Check sheet for the drawn part. Datum: minimum x, y, z corner. Units: mm. A direction names the side the tool comes from. Round coordinates to 2 decimals unless told otherwise and drop trailing zeros. Order: outer loops, then holes, each group sorted by start corner. A loop starts at its lowest first (then second) coordinate and runs counter-clockwise, first axis right, second up. Notation, with made-up numbers: (61.5, 15.5) -> (95.5, 15.5) arc R20 cw to (95.5, 36.5) -> close; hole circle Ø7 at (11.25, -2). An arc over 180 degrees is marked (long way). Answer as a JSON object with one key per item and string values. Group by question number.
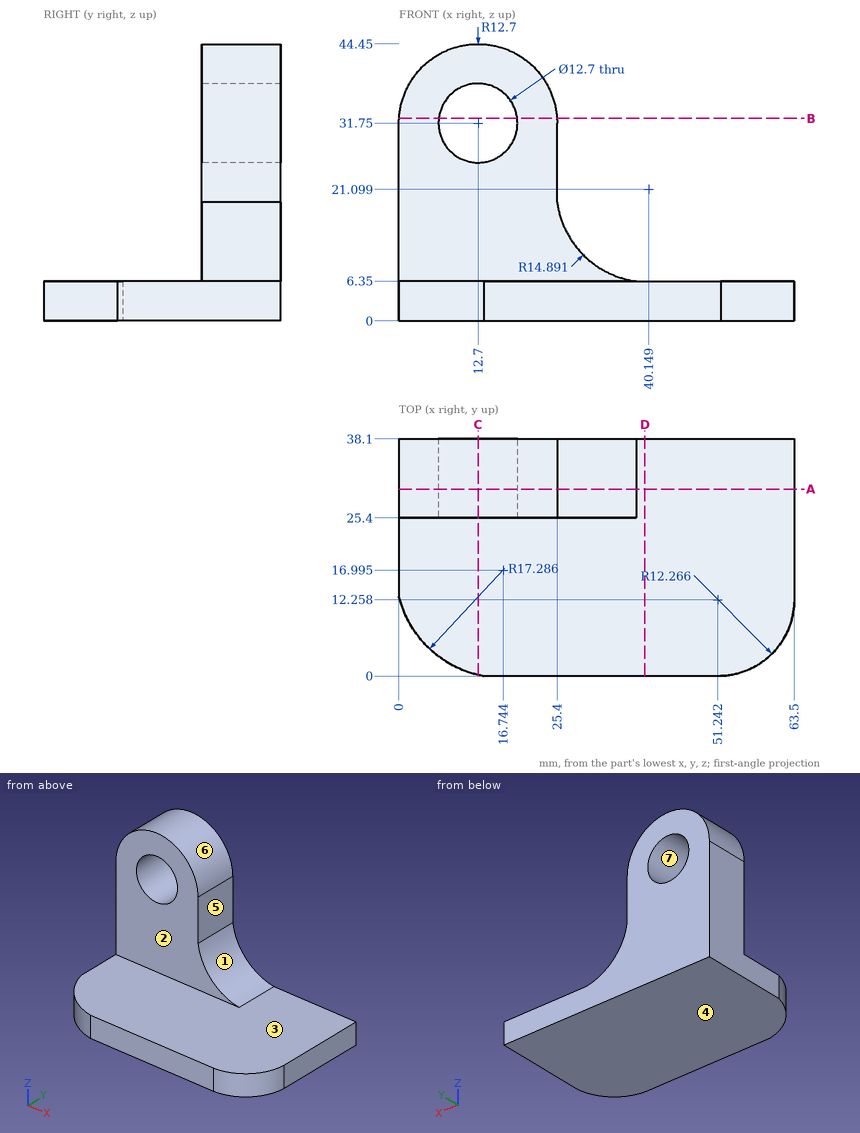
Item 1: Depth check by flat-ended pin: pin 1 Ø20.5 at (x, z) = (12.7, 31.75) entering from +Y; pin 2 Ø3 at (x, z) = (7.5, 31.5) entering from -Y; pin 3 Ø11.5 at (x, y) = (34, 18) entering from +Z; pin 4 Ø14 at (y, z) = (34, 26.5) entering from +X. Enter the tip coordinate at first touch or a pass-through.
Item 2: Mould release check, pull along Z, two halves, no side actions. Record for the marked faces 4, 5, 6 and 7: pulls with the +Z half, pulls with the -Z half, needs draft (parallel to the pull), parting line crosses it, or undercut.
Item 3: Thickness scan on L1, parallel to Z at x = 12.7, y = 29.5; L2, parallel to Z at x = 57, y = 30; L3, parallel to X at y = 30, z = 31 (1 decimal). Record the ranges inside material, lowest first.
Item 4: Sectioned sample at D-D, the plane x = 39.5. Enter the section's corners in (y, z), then the cut area to 3 significant figures.
Item 5: Sectioned sample at A-A, the plane y = 30. Enter the section's corners in (x, z), then the cut area to 3 significant figures.
Item 6: Set-up check for the marked faces 1, 2 and 3: record each of +Z, -Z, +X, -X, +Y, -Y from which the full face is reachable in a straight line by a thin tool's end or side.
Item 7: Sectioned sample at C-C, the plane x = 12.7. Enter the section's corners in (y, z), then the cut area to 3 significant figures.
Item 8: Sectioned sample at B-B, the plane z = 32.5. Enter the section's corners in (x, y) (1 decimal), then the cut area to 3 significant figures.
Result:
{
 "1": {"pin 1": "stops at y = 38.1", "pin 2": "stops at y = 25.4", "pin 3": "stops at z = 6.35", "pin 4": "stops at x = 25.4"},
 "2": {"face 4": "pulls with the -Z half", "face 5": "needs draft", "face 6": "pulls with the +Z half", "face 7": "undercut"},
 "3": {"L1": "z = 0 to 25.4, 38.1 to 44.45", "L2": "z = 0 to 6.35", "L3": "x = 0 to 6.4, 19 to 25.4"},
 "4": {"outline": "(0, 0) -> (38.1, 0) -> (38.1, 6.35) -> (0, 6.35) -> close", "area": "242 mm2"},
 "5": {"outline": "(0, 0) -> (63.5, 0) -> (63.5, 6.35) -> (38.1, 6.35) arc R14.89 cw to (25.4, 19.05) -> (25.4, 31.75) arc R12.7 ccw to (0, 31.75) -> close; hole circle Ø12.7 at (12.7, 31.75)", "area": "1,220 mm2"},
 "6": {"face 1": "+Z, +X, +Y, -Y", "face 2": "+Z, +X, -X, -Y", "face 3": "+Z, +X, -Y"},
 "7": {"outline": "(0.19, 0) -> (38.1, 0) -> (38.1, 25.4) -> (25.4, 25.4) -> (25.4, 6.35) -> (0.19, 6.35) -> close; (25.4, 38.1) -> (38.1, 38.1) -> (38.1, 44.45) -> (25.4, 44.45) -> close", "area": "563 mm2"},
 "8": {"outline": "(0, 25.4) -> (6.4, 25.4) -> (6.4, 38.1) -> (0, 38.1) -> close; (19, 25.4) -> (25.4, 25.4) -> (25.4, 38.1) -> (19, 38.1) -> close", "area": "162 mm2"}
}
